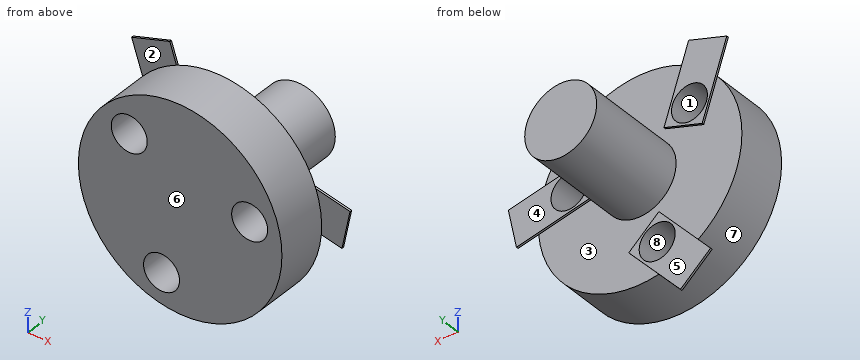
Autodesk Inventor part; units mm, degrees
ref_plane "YZ Plane" through (0, 0, 0) normal (1, 0, 0) x (0, 1, 0)
ref_plane "XZ Plane" through (0, 0, 0) normal (0, 1, 0) x (-1, 0, 0)
ref_plane "XY Plane" through (0, 0, 0) normal (0, 0, 1) x (1, 0, 0)
sketch "Sketch1" plane through (0, 0, 0) normal (0, 1, 0) x (-1, 0, 0)
  circle A0 centre (0, 0) radius 12.7
  dimension "d0" = 25.4
extrude "Extrusion1" add sketch "Sketch1" along normal blind 6.35
sketch "Sketch2" plane through (0, 6.35, 0) normal (0, 1, 0) x (1, 0, 0)
  line L0 (0, 0) -> (-6.35, 0)
  circle A0 centre (-6.35, -6.35) radius 2.2451
  line L1 (-3.175, -4.7625) -> (-7.9375, -3.175)
  line L2 (-7.9375, -3.175) -> (-11.0117, -12.3975)
  line L3 (-3.175, -4.7625) -> (-6.2492, -13.985)
  line L4 (-11.0117, -12.3975) -> (-6.2492, -13.985)
  circle A1 centre (8.6743, -2.3243) radius 2.2451
  line L5 (6.7184, -5.2866) -> (16.2423, -3.3376)
  line L6 (16.2423, -3.3376) -> (15.2359, 1.5806)
  line L7 (5.7119, -0.3684) -> (15.2359, 1.5806)
  line L8 (5.7119, -0.3684) -> (6.7184, -5.2866)
  circle A2 centre (-2.3243, 8.6743) radius 2.2451
  line L9 (1.2191, 8.4616) -> (-5.2307, 15.7351)
  line L10 (-5.2307, 15.7351) -> (-8.9867, 12.4044)
  line L11 (-2.5369, 5.1309) -> (-8.9867, 12.4044)
  line L12 (-2.5369, 5.1309) -> (1.2191, 8.4616)
  dimension "d5" = 360
extrude "Extrusion2" add sketch "Sketch2" along normal blind 0.254
sketch "Sketch3" plane through (-6.35, 6.35, 6.35) normal (0, 1, 0) x (1, 0, 0)
  point P0 (6.35, 6.35)
sketch "Sketch4" plane through (0, 6.35, 0) normal (0, 1, 0) x (1, 0, 0)
  circle A0 centre (-6.35, -6.35) radius 2.2451
  circle A1 centre (8.6743, -2.3243) radius 2.2451
  circle A2 centre (-2.3243, 8.6743) radius 2.2451
  point P0 (0, 0)
  dimension "d11" = 360
extrude "Extrusion3" cut sketch "Sketch4" against normal blind 12.7
sketch "Sketch5" plane through (0, 6.35, 0) normal (0, 1, 0) x (1, 0, 0)
  circle A0 centre (0, 0) radius 4.4901
extrude "Extrusion4" add sketch "Sketch5" along normal blind 12.7
properties part number "hand_shaft"
Model file for the job. Use its own axes, mm. Face numbers are marked on the shaded views. A direction names the side the tool comes from. Give positions to 0.01 mm unless a question says otherwise; leave off trailing zeros. Order: outer loops, then holes, each group sorted by start corner. A loop starts at its lowest first (then second) coordinate and runs counter-clockwise, first axis right, second up. Notation, with made-up numbers: (30.5, 2.5) -> (59.5, 2.5) arc R18 ccw to (59.5, 9.5) -> close; hole circle Ø6 at (27, 58.5). An arc over 180 degrees is marked (long way). Use CSV: the item, a comma, the result in double quotes.
1. Band-saw the part on D-D, the plane y = 11. Give the cut face in (x, z).
Outcome:
outline,"circle Ø8.98 at (0, 0)"
2. Drop flat-ended pins along their axis: pin 1 (5 mm diameter, centred on x = -6, z = -8.5, fed in from +Y); pin 2 (6 mm diameter, centred on y = 8, z = -12.5, fed in from -X); pin 3 (2.5 mm diameter, centred on x = -4.5, z = -14, fed in from -Y). Give the stop position or say it passes through.
Outcome:
pin 1,"y = 6.6"
pin 2,"x = -8.99"
pin 3,"y = 6.35"
3. Band-saw the part on A-A, the plane x = -1.25. Give the cut face in (y, z).
Outcome:
outline,"(0, -12.64) -> (6.35, -12.64) -> (6.35, -11.25) -> (6.6, -11.25) -> (6.6, -10.65) -> (0, -10.65) -> close; (0, -6.7) -> (6.6, -6.7) -> (6.6, -6.27) -> (6.35, -6.27) -> (6.35, -4.31) -> (19.05, -4.31) -> (19.05, 4.31) -> (6.35, 4.31) -> (6.35, 12.64) -> (0, 12.64) -> close"
4. Band-saw the part on C-C, the plane z = -3. Give the cut face in (x, y).
Outcome:
outline,"(-12.34, 0) -> (12.34, 0) -> (12.34, 6.35) -> (3.34, 6.35) -> (3.34, 19.05) -> (-3.34, 19.05) -> (-3.34, 6.35) -> (-12.34, 6.35) -> close"
5. Drill centre lines: line 1 along X through (y, z) = (3.25, 3.5); line 2 along X through (y, z) = (5.5, 2.5); line 3 along Y through (x, z) = (-2.25, -4.75). Where is each one in solid material? Low to high. Write a range as from..to.
Outcome:
line 1,"-12.21..6.76, 10.59..12.21"
line 2,"-12.45..6.44, 10.91..12.45"
line 3,"0..6.35"
6. Mould opens along Z. For the marked faces 6, 7 and 8 say: +Z half, -Z half, draft (parallel to the pull), parting line (faces both ways), or undercut.
Outcome:
face 6,"draft"
face 7,"parting line"
face 8,"undercut"
7. Band-saw the part on B-B, the plane z = 6.35. Give the cut face in (x, y), then the cut area to 3 significant figures.
Outcome:
outline,"(-11, 0) -> (-8.6, 0) -> (-8.6, 6.6) -> (-9, 6.6) -> (-9, 6.35) -> (-11, 6.35) -> close; (-4.1, 0) -> (11, 0) -> (11, 6.35) -> (-3.7, 6.35) -> (-3.7, 6.6) -> (-4.1, 6.6) -> close"
area,"111 mm²"
8. 3-axis set-ups, long thin cutter, end or side, ignore diameter. For the marked faces 1, 2, 3, 4 and 5: which of +Z, -Z, +X, -X, +Y, -Y reach the whole face in a straight line?
Outcome:
face 1,"+Y, -Y"
face 2,"+Z, -X, -Y"
face 3,"+Y"
face 4,"+Z, -Z, +X, +Y"
face 5,"-Z, +X, -X, +Y"
